Here's how the part is built. I have some questions about the finished solid (model axes, mm). A direction names the side the tool comes from. Give positions to 0.01 mm unless a question says otherwise; leave off trailing zeros. Order: outer loops, then holes, each group sorted by start corner. A loop starts at its lowest first (then second) coordinate and runs counter-clockwise, first axis right, second up.
from build123d import *

# Parameters (mm, degrees)
F0_W     = 26
F0_H     = 26
F1_DEPTH = 13
F2_R     = 1
F3_R     = 5
F4_R     = 7
F5_DEPTH = 17
F6_R     = 0.5


with BuildPart() as f1:
    # F0 (on Top) → F1 (new body)
    with BuildSketch(Plane.XY):
        with Locations((-41.661934, 26.971549)):
            Rectangle(F0_W, F0_H)
    extrude(amount=F1_DEPTH)

    # F2
    f2_edges = [f1.edges().sort_by_distance(p)[0] for p in [
        (-28.661934, 26.971549, 0),
        (-41.661934, 39.971549, 0),
        (-54.661934, 26.971549, 0),
        (-41.661934, 13.971549, 0),
    ]]
    fillet(f2_edges, radius=F2_R)

    # F3
    f3_edges = [f1.edges().sort_by_distance(p)[0] for p in [
        (-41.661934, 39.971549, 13),
        (-54.661934, 26.971549, 13),
        (-41.661934, 13.971549, 13),
        (-28.661934, 26.971549, 13),
    ]]
    fillet(f3_edges, radius=F3_R)

    # F4 (on face) → F5 (join)
    with BuildSketch(Plane.XY.offset(13)):
        with Locations((-41.661934, 26.971549)):
            Circle(F4_R)
    extrude(amount=F5_DEPTH)

    # F6
    f6_edges = [f1.edges().sort_by_distance(p)[0] for p in [
        (-48.661934, 26.971549, 30),
    ]]
    fillet(f6_edges, radius=F6_R)


solid = f1.part
Q1. If we section it at D-D on z = 24.5: List the corners of the cut face in (x, y) for me, plus the area to 3 significant figures.
Filled sheet:
outline: circle Ø14 at (-41.66, 26.97)
area: 154 mm2
Q2. If we section it at B-B on x = -32.75: List the corners of the cut face in (y, z) for me.
Filled sheet:
outline: (13.97, 1) arc R1 ccw to (14.97, 0) - (38.97, 0) arc R1 ccw to (39.97, 1) - (39.97, 8) arc R5 ccw to (35.88, 12.92) - (18.06, 12.92) arc R5 ccw to (13.97, 8) - close
Q3. If we section it at C-C on z = 10.5: List the corners of the cut face in (x, y) for me, plus the area to 3 significant figures.
Filled sheet:
outline: (-53.99, 14.64) - (-29.33, 14.64) - (-29.33, 39.3) - (-53.99, 39.3) - close
area: 608 mm2
Q4. If we section it at A-A on y = 19.5: List the corners of the cut face in (x, z) for me.
Filled sheet:
outline: (-54.66, 1) arc R1 ccw to (-53.66, 0) - (-29.66, 0) arc R1 ccw to (-28.66, 1) - (-28.66, 8) arc R5 ccw to (-33.66, 13) - (-49.66, 13) arc R5 ccw to (-54.66, 8) - close
Q5. For faces 1 (the face through (-42, 27, 30)), 2 (the face through (-48.655, 27.279, 21.134)), which set-ups out of +Z, -Z, +X, -X, +Y, -Y let a thin tool reach every point of the face, with its end or its side?
Filled sheet:
face 1: +Z, +X, -X, +Y, -Y
face 2: +Z
Q6. I'm going to push flat-ended pins straight in: P1, Ø10, axis at x = -37, z = 16.5, coming from the -Y side; P2, Ø5, axis at y = 22.5, z = 18, coming from the -X side; P3, Ø12, axis at x = -36.5, z = 25, coming from the -Y side. Where does each tip first touch, or does it pass through?
Filled sheet:
P1: stops at y = 15.4
P2: stops at x = -48.38
P3: stops at y = 19.97
Q7. I need wall thicknesses on L1, parallel to Z at x = -37, y = 20; L2, parallel to Y at x = -41, z = 17.75; L3, parallel to Z at x = -43, y = 15.5. Which ranges of each line are inside material? Lowest first, please.
Filled sheet:
L1: z = 0 to 13
L2: y = 20 to 33.94
L3: z = 0 to 11.6
